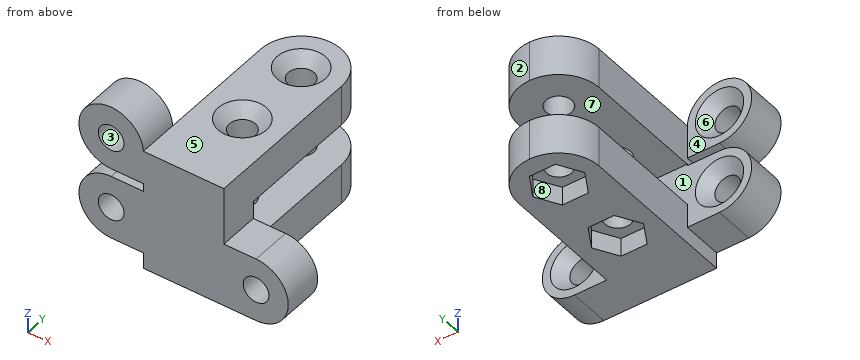
Autodesk Inventor part; units mm, degrees
ref_plane "РабПлоскость1" through (0, 0, -7.6) normal (0, 0, -1) x (-1, 0, 0)
ref_plane "РабПлоскость2" through (0, 0, -12.9) normal (0, 0, -1) x (-1, 0, 0)
ref_plane "YZ Plane" through (0, 0, 0) normal (1, 0, 0) x (0, 1, 0)
sketch "Эскиз3" plane through (0, 0, 0) normal (0, 1, 0) x (-1, 0, 0)
  line L0 (0, 0) -> (10, 0)
  line L1 (10, 0) -> (10, -5)
  line L2 (10, -5) -> (0, -5)
  line L3 (0, -5) -> (0, 0)
  dimension "d6" = 10
  dimension "d7" = 5
extrude "Выдавливание2" add sketch "Эскиз3" along normal blind 20
fillet "Сопряжение1" radius 5 2 edges at (0, 20, -2.5) (-10, 20, -2.5)
ref_plane "РабПлоскость1" through (0, 0, -7.6) normal (0, 0, -1) x (-1, 0, 0)
mirror "Зеркальное отражение1" about plane through (0, 0, -7.6) normal (0, 0, -1)
ref_plane "РабПлоскость2" through (0, 0, -12.9) normal (0, 0, -1) x (-1, 0, 0)
sketch "Эскиз5" plane through (-10, 0, 0) normal (0, 0, 1) x (1, 0, 0)
  arc A0 (10, 15) -> (0, 15) centre (5, 15) ccw
  line L0 (5, 15) -> (5, 5)
  dimension "d23" = 10
hole "Отверстие1" at (-5, 15, 0) at (-5, 5, 0) direction (0, 0, -1) diameter 3.2 depth 12.9 countersink diameter 6 countersink angle 90
sketch "Эскиз6" plane through (-10, 0, -15.2) normal (0, 0, 1) x (1, 0, 0)
  circle A0 centre (5, 15) radius 1.6
  circle A1 centre (5, 5) radius 1.6
  line L0 (6.6166, 17.8) -> (8.2332, 15)
  line L1 (8.2332, 15) -> (6.6166, 12.2)
  line L2 (6.6166, 12.2) -> (3.3834, 12.2)
  line L3 (3.3834, 12.2) -> (1.7668, 15)
  line L4 (1.7668, 15) -> (3.3834, 17.8)
  line L5 (3.3834, 17.8) -> (6.6166, 17.8)
  line L6 (6.6166, 7.8) -> (8.2332, 5)
  line L7 (8.2332, 5) -> (6.6166, 2.2)
  line L8 (6.6166, 2.2) -> (3.3834, 2.2)
  line L9 (3.3834, 2.2) -> (1.7668, 5)
  line L10 (1.7668, 5) -> (3.3834, 7.8)
  line L11 (3.3834, 7.8) -> (6.6166, 7.8)
  point P0 (10, 0)
  dimension "d24" = 5.6
  dimension "d25" = 5.6
extrude "Выдавливание3" cut sketch "Эскиз6" along normal up to surface (2.3 mm away) contours A0 | A1 | L0 L1 L2 L3 L4 L5 | L6 L7 L8 L9 L10 L11
sketch "Эскиз9" plane through (-10, 0, -15.2) normal (0, -1, 0) x (1, 0, 0)
  line L0 (0, 5) -> (0, 0)
  line L1 (10, 15.2) -> (0, 15.2)
  line L2 (0, 15.2) -> (0, 0)
  line L3 (0, 0) -> (10, 0)
  line L4 (10, 0) -> (10, 15.2)
extrude "Выдавливание5" add sketch "Эскиз9" along normal blind 5
sketch "Эскиз11" plane through (-10, -5, -15.2) normal (0, -1, 0) x (1, 0, 0)
  line L0 (0, 15.2) -> (0, 0)
  line L1 (0, 0) -> (10, 0)
  line L2 (10, 0) -> (10, 15.2)
  line L3 (10, 15.2) -> (0, 15.2)
  line L4 (10, 0) -> (18, 0)
  line L5 (18, 0) -> (18, 8)
  line L6 (18, 8) -> (10, 8)
  line L7 (10, 8) -> (10, 0)
  line L8 (0, 0) -> (0, 2)
  line L9 (0, 5) -> (0, 0)
  line L10 (0, 2) -> (-8, 2)
  line L11 (-8, 2) -> (-8, 10)
  line L12 (-8, 10) -> (0, 10)
  line L13 (0, 10) -> (0, 2)
  line L14 (0, 10) -> (0, 11)
  line L15 (0, 10.2) -> (0, 15.2)
  line L16 (0, 11) -> (-8, 11)
  line L17 (-8, 11) -> (-8, 19)
  line L18 (-8, 19) -> (0, 19)
  line L19 (0, 19) -> (0, 11)
  point P0 (0, 2)
  dimension "d75" = 8
  dimension "d76" = 8
  dimension "d77" = 2
  dimension "d78" = 8
  dimension "d79" = 8
  dimension "d80" = 1
  dimension "d81" = 8
  dimension "d82" = 8
extrude "Выдавливание6" add sketch "Эскиз11" against normal blind 5 contours L0 L16 L17 L18 L19 | L6 L5 L4 L2 | L0 L10 L11 L12
sketch "Эскиз12" plane through (-10, 0, -15.2) normal (0, 1, 0) x (1, 0, 0)
  line L0 (10, -10.2) -> (0, -10.2)
  line L1 (10, -8) -> (10, -10.2)
  line L2 (10, -8) -> (18, -8)
  line L3 (18, -8) -> (18, 0)
  line L4 (18, 0) -> (10, 0)
  line L5 (10, -5) -> (10, 0)
  line L6 (10, -5) -> (0, -5)
  line L7 (0, -2) -> (0, -5)
  line L8 (0, -2) -> (-8, -2)
  line L9 (-8, -2) -> (-8, -10)
  line L10 (-8, -10) -> (0, -10)
  line L11 (0, -10.2) -> (0, -10)
  line L12 (0, -11) -> (-8, -11)
  line L13 (-8, -11) -> (-8, -19)
  line L14 (-8, -19) -> (0, -19)
  line L15 (0, -19) -> (0, -15.2)
  line L16 (0, -11) -> (0, -15.2)
  line L17 (0, -2) -> (-8, -2)
  line L18 (-4, -2) -> (-4, -10)
  line L19 (0, -11) -> (-8, -11)
  line L20 (-4, -11) -> (-4, -19)
  line L21 (18, 0) -> (10, 0)
  line L22 (14, 0) -> (14, -8)
  point P0 (10, -15.2)
  point P1 (14, -4)
  point P2 (-4, -6)
  point P3 (-4, -15)
hole "Отверстие4" at (-14, 0, -9.2) at (4, 0, -11.2) at (-14, 0, -0.2) direction (0, -1, 0) diameter 3.2 end through all countersink diameter 6 countersink angle 90
fillet "Сопряжение2" radius 4 7 edges at (8, -2.5, -15.2) (8, -2.5, -7.2) (-18, -2.5, -13.2) (-18, -2.5, -5.2) (-18, -2.5, -4.2) (-18, -2.5, 3.8) (-10, -2.5, 3.8)
equation "\"d25\" = d24"
properties part number "Крепление камеры к корпусу"
Part model, mm, in its own coordinate system. Face numbers are marked on the shaded views. A direction names the side the tool comes from. Coordinates: 2 decimals unless noted, no trailing zeros. Write each loop counter-clockwise with the first axis right and the second up, starting at its lowest first coordinate (ties: lowest second). Pieces come first, ordered by that corner, then holes.
Item 1: Slice it at B-B (y = -0.75). Write the cut outline in (x, z) (3 decimals), and give its area (3 significant figures).
Item 2: Slice it at A-A (y = 9.5). Write the cut outline in (x, z).
Item 3: Slice it at C-C (x = -0.75). Write the cut outline in (y, z).
Item 4: Which spindle directions (+Z, -Z, +X, -X, +Y, -Y) get a long thin tool onto all of the face, cutting with end or side? Do the marked faces 4, 5, 6, 7 and 8. Say none if no direction does.
Item 5: Pin check, flat tips, straight feed: pin 1 (4 mm diameter, centred on x = -13, z = 1, fed in from +Y); pin 2 (3 mm diameter, centred on x = -5, y = 5, fed in from +Z); pin 3 (12 mm diameter, centred on x = -5, y = 5, fed in from +Z); pin 4 (1 mm diameter, centred on y = -2.5, z = -5, fed in from -X). Stop position of each tip, or through.
Item 6: Probe line 1 (Z direction, x = -14, y = -4.1); line 2 (Y direction, x = -5, z = -4.05); line 3 (X direction, y = -3.5, z = -0.2). List the from-to ranges inside material, lowest first.
Item 7: Mould opens along X. For the marked faces 1, 2 and 3 say: released by +X, released by -X, zero draft, split by the parting line, or undercut.
Results found:
1. outline: (-14, -13.2) - (-10, -13.2) - (-10, -15.2) - (4, -15.2) arc R4 ccw to (4, -7.2) - (0, -7.2) - (0, 0) - (-10.005, 0) arc R4 ccw (long way) to (-14, -4.2) - (-10, -4.2) - (-10, -5.2) - (-14, -5.2) arc R4 ccw to start; hole circle Ø4.5 at (-14, -9.2); hole circle Ø4.5 at (-14, -0.2); hole circle Ø4.5 at (4, -11.2)
1. area: 272 mm2
2. outline: (-10, -15.2) - (0, -15.2) - (0, -10.2) - (-10, -10.2) - close; (-10, -5) - (0, -5) - (0, 0) - (-10, 0) - close
3. outline: (-5, -15.2) - (17.63, -15.2) - (17.63, -10.2) - (0, -10.2) - (0, -5) - (17.63, -5) - (17.63, 0) - (-5, 0) - close
4. face 4: +Z, -Z, -X, +Y
4. face 5: +Z, +X, +Y, -Y
4. face 6: +Y
4. face 7: +X, -X, +Y
4. face 8: -Z
5. pin 1: stops at y = 0
5. pin 2: passes through
5. pin 3: stops at z = 0
5. pin 4: stops at x = -15.52
6. line 1: z = -13.2 to -10.8, -7.6 to -5.2, -4.2 to -1.8, 1.4 to 3.8
6. line 2: y = -5 to 3.4, 6.6 to 13.4, 16.6 to 20
6. line 3: x = -18 to -15.6, -12.4 to 0
7. face 1: zero draft
7. face 2: released by +X
7. face 3: undercut
